from build123d import *

# Parameters (mm, degrees)
BOSS_EXTRUDE1_DEPTH      = 42
BOSS_EXTRUDE1_DEPTH_BACK = 42
BOSS_EXTRUDE2_DEPTH      = 34
BOSS_EXTRUDE2_DEPTH_BACK = 34
SKETCH1_3_W              = 50
SKETCH1_3_H              = 50
SKETCH2_W                = 48
SKETCH2_H                = 30
CUT_EXTRUDE1_DEPTH       = 135.029847422
SKETCH3_R                = 16
CUT_EXTRUDE2_DEPTH       = 119.697093477


with BuildPart() as part:
    # Sketch1 → Boss-Extrude1 (new, two sides: drawn at the far end of the back side and taken through both)
    with BuildSketch(Plane.XY.offset(-BOSS_EXTRUDE1_DEPTH_BACK)):
        Polygon((-30, 0), (-30, 8), (30, 8), (30, 0), (65, 0), (65, 12), (25, 35), (25, 40), (-25, 40), (-25, 35), (-65, 12), (-65, 0), align=None)
    extrude(amount=BOSS_EXTRUDE1_DEPTH + BOSS_EXTRUDE1_DEPTH_BACK)

    # Sketch1<3> → Boss-Extrude2 (add, two sides: drawn at the far end of the back side and taken through both)
    with BuildSketch(Plane.XY.offset(-BOSS_EXTRUDE2_DEPTH_BACK)):
        with Locations((0, 65)):
            Rectangle(SKETCH1_3_W, SKETCH1_3_H)
    extrude(amount=BOSS_EXTRUDE2_DEPTH + BOSS_EXTRUDE2_DEPTH_BACK)

    # Sketch2 → Cut-Extrude1 (cut, through all)
    with BuildSketch(Plane(origin=(25, 0, 0), x_dir=(0, 0, -1), z_dir=(1, 0, 0))):
        with Locations((0, 65)):
            Rectangle(SKETCH2_W, SKETCH2_H)
    extrude(amount=-CUT_EXTRUDE1_DEPTH, mode=Mode.SUBTRACT)

    # Sketch3 → Cut-Extrude2 (cut, through all)
    with BuildSketch(Plane.XZ):
        Circle(SKETCH3_R)
        Polygon((-35, 29), (-57, 0), (-35, -29), align=None)
        Polygon((35, -29), (35, 29), (57, 0), align=None)
    extrude(amount=-CUT_EXTRUDE2_DEPTH, mode=Mode.SUBTRACT)


solid = part.part
Verification items for the finished model (mm, model axes). A direction names the side the tool comes from. Coordinates: 2 decimals unless noted, no trailing zeros. Order: outer loops, then holes, each group sorted by start corner. A loop starts at its lowest first (then second) coordinate and runs counter-clockwise, first axis right, second up.
1. Scan lines: line 1 (Z direction, x = 0, y = 42.5); line 2 (X direction, y = 22, z = 24); line 3 (Z direction, x = 0, y = 19). Record each from-to range of solid material in increasing order.
Results found:
line 1: z = -34 to -16, 16 to 34
line 2: x = -47.61 to -38.79, -35 to 35, 38.79 to 47.61
line 3: z = -42 to -16, 16 to 42
2. Release check for a two-part mould opening along Z. For faces 1 (the face through (0, 65, -34)), 2 (the face through (-46.15, 11.17, -14.3)), 3 (the face through (-35, 14, 0)), 4 (the face through (-52, 0, -10)) record: +Z half, -Z half, draft (parallel to the pull), parting line (faces both ways), or undercut.
Results found:
face 1: -Z half
face 2: undercut
face 3: undercut
face 4: draft
3. Set-up check for faces 5 (the face through (-30, 4, -1)), 6 (the face through (45.85, 11.17, 14.7)), 7 (the face through (0.4, 50, 16.3)): record each of +Z, -Z, +X, -X, +Y, -Y from which the full face is reachable in a straight line by a thin tool's end or side.
Results found:
face 5: +Z, -Z, -Y
face 6: +Y, -Y
face 7: +X, -X
4. Sectioned sample at B-B, the plane y = 64. Record the cut outline in (x, z).
Results found:
outline: (-25, -34) - (25, -34) - (25, -24) - (-25, -24) - close; (-25, 24) - (25, 24) - (25, 34) - (-25, 34) - close
5. Go/stop test with flat-tipped pins: pin 1 Ø25 at (x, y) = (9, 66.5) entering from -Z; pin 2 Ø1.5 at (y, z) = (36, -2) entering from +X; pin 3 Ø16.5 at (y, z) = (57, -1) entering from -X; pin 4 Ø24 at (x, z) = (5.5, 12) entering from +Y. Record where each tip stops, or that it passes through.
Results found:
pin 1: stops at z = -34
pin 2: stops at x = 25
pin 3: stops at x = -25
pin 4: stops at y = 90
6. Sectioned sample at C-C, the plane z = -35.5. Record the cut outline in (x, y), and give its area (3 significant figures).
Results found:
outline: (-65, 0) - (-30, 0) - (-30, 8) - (30, 8) - (30, 0) - (65, 0) - (65, 12) - (25, 35) - (25, 40) - (-25, 40) - (-25, 35) - (-65, 12) - close
area: 3,400 mm2
7. Sectioned sample at D-D, the plane x = 0. Record the cut outline in (y, z).
Results found:
outline: (8, -42) - (40, -42) - (40, -34) - (90, -34) - (90, -16) - (80, -16) - (80, -24) - (50, -24) - (50, -16) - (8, -16) - close; (8, 16) - (50, 16) - (50, 24) - (80, 24) - (80, 16) - (90, 16) - (90, 34) - (40, 34) - (40, 42) - (8, 42) - close
8. Sectioned sample at A-A, the plane x = 19.5. Record the cut outline in (y, z).
Results found:
outline: (8, -42) - (40, -42) - (40, -34) - (90, -34) - (90, 34) - (40, 34) - (40, 42) - (8, 42) - close; hole (50, -24) - (80, -24) - (80, 24) - (50, 24) - close
